```python
from build123d import *

# Parameters (mm, degrees)
SKETCH1_W           = 91
SKETCH1_H           = 104
SKETCH1_W_2         = 87
SKETCH1_H_2         = 100
BOSS_EXTRUDE1_DEPTH = 12
SKETCH2_W           = 91
SKETCH2_H           = 104
BOSS_EXTRUDE2_DEPTH = 2
SKETCH3_R           = 3.5
BOSS_EXTRUDE3_DEPTH = 12
SKETCH6_W           = 8
SKETCH6_H           = 5
BOSS_EXTRUDE4_DEPTH = 14
CUT_EXTRUDE1_REACH  = 141.879
SKETCH4_R           = 1.5
SKETCH7_R           = 2.9
CUT_EXTRUDE2_DEPTH  = 8
SKETCH8_W           = 33
SKETCH8_H           = 2
CUT_EXTRUDE3_DEPTH  = 1.3
SKETCH9_W           = 87.4
SKETCH9_H           = 100.4
SKETCH9_W_2         = 87
SKETCH9_H_2         = 100
CUT_EXTRUDE4_DEPTH  = 0.2
SKETCH10_W          = 6
SKETCH10_H          = 10
BOSS_EXTRUDE7_DEPTH = 5
CUT_EXTRUDE5_REACH  = 143.23
SKETCH11_R          = 0.75
SKETCH12_W          = 37
SKETCH12_H          = 7.6
CUT_EXTRUDE6_DEPTH  = 7
CUT_EXTRUDE7_REACH  = 142.975
SKETCH13_W          = 72
SKETCH13_H          = 7.6
FILLET1_R           = 10
FILLET2_R           = 2
SKETCH14_W          = 10
SKETCH14_H          = 4
CUT_EXTRUDE8_DEPTH  = 0.5


with BuildPart() as part:
    # Sketch1 → Boss-Extrude1 (new body)
    with BuildSketch(Plane(origin=(0, 0, 0), x_dir=(1, 0, 0), z_dir=(0, 1, 0))):
        with Locations((43.5, 50)):
            Rectangle(SKETCH1_W, SKETCH1_H)
        with Locations((43.5, 50)):
            Rectangle(SKETCH1_W_2, SKETCH1_H_2, mode=Mode.SUBTRACT)
    extrude(amount=-BOSS_EXTRUDE1_DEPTH)

    # Sketch2 → Boss-Extrude2 (add)
    with BuildSketch(Plane(origin=(0, 0, 0), x_dir=(1, 0, 0), z_dir=(0, 1, 0))):
        with Locations((43.5, 50)):
            Rectangle(SKETCH2_W, SKETCH2_H)
    extrude(amount=BOSS_EXTRUDE2_DEPTH)

    # Sketch3 → Boss-Extrude3 (add)
    with BuildSketch(Plane.XZ):
        with Locations(Location((5, -5, 0), (0, 0, 90))):
            Circle(SKETCH3_R)
        with Locations(Location((5, -95, 0), (0, 0, 90))):
            Circle(SKETCH3_R)
        with Locations(Location((50.38, -8.15, 0), (0, 0, 90))):
            Circle(SKETCH3_R)
        with Locations(Location((25, -50, 0), (0, 0, 90))):
            Circle(SKETCH3_R)
    extrude(amount=BOSS_EXTRUDE3_DEPTH)

    # Sketch6 → Boss-Extrude4 (add, through all)
    with BuildSketch(Plane(origin=(0, 2, 0), x_dir=(1, 0, 0), z_dir=(0, 1, 0))):
        with Locations((85, 104.5)):
            Rectangle(SKETCH6_W, SKETCH6_H)
        with Locations((85, -4.5)):
            Rectangle(SKETCH6_W, SKETCH6_H)
    extrude(amount=-BOSS_EXTRUDE4_DEPTH)

    # Sketch4 → Cut-Extrude1 (cut, up to next)
    with BuildSketch(Plane(origin=(0, 2, 0), x_dir=(1, 0, 0), z_dir=(0, 1, 0)), mode=Mode.PRIVATE) as cut_extrude1_sk1:
        with Locations(Location((5, 5, 0), (0, 0, 270))):
            Circle(SKETCH4_R)
    cut_extrude1_tool1 = extrude(cut_extrude1_sk1.sketch, amount=-CUT_EXTRUDE1_REACH, mode=Mode.PRIVATE) & part.part
    # Sketch4 → Cut-Extrude1 (cut, up to next)
    with BuildSketch(Plane(origin=(0, 2, 0), x_dir=(1, 0, 0), z_dir=(0, 1, 0)), mode=Mode.PRIVATE) as cut_extrude1_sk2:
        with Locations(Location((5, 95, 0), (0, 0, 270))):
            Circle(SKETCH4_R)
    cut_extrude1_tool2 = extrude(cut_extrude1_sk2.sketch, amount=-CUT_EXTRUDE1_REACH, mode=Mode.PRIVATE) & part.part
    # Sketch4 → Cut-Extrude1 (cut, up to next)
    with BuildSketch(Plane(origin=(0, 2, 0), x_dir=(1, 0, 0), z_dir=(0, 1, 0)), mode=Mode.PRIVATE) as cut_extrude1_sk3:
        with Locations(Location((50.38, 8.15, 0), (0, 0, 270))):
            Circle(SKETCH4_R)
    cut_extrude1_tool3 = extrude(cut_extrude1_sk3.sketch, amount=-CUT_EXTRUDE1_REACH, mode=Mode.PRIVATE) & part.part
    # Sketch4 → Cut-Extrude1 (cut, up to next)
    with BuildSketch(Plane(origin=(0, 2, 0), x_dir=(1, 0, 0), z_dir=(0, 1, 0)), mode=Mode.PRIVATE) as cut_extrude1_sk4:
        with Locations(Location((25, 50, 0), (0, 0, 270))):
            Circle(SKETCH4_R)
    cut_extrude1_tool4 = extrude(cut_extrude1_sk4.sketch, amount=-CUT_EXTRUDE1_REACH, mode=Mode.PRIVATE) & part.part
    # Sketch4 → Cut-Extrude1 (cut, up to next)
    with BuildSketch(Plane(origin=(0, 2, 0), x_dir=(1, 0, 0), z_dir=(0, 1, 0)), mode=Mode.PRIVATE) as cut_extrude1_sk5:
        with Locations(Location((85, 103.5, 0), (0, 0, 270))):
            Circle(SKETCH4_R)
    cut_extrude1_tool5 = extrude(cut_extrude1_sk5.sketch, amount=-CUT_EXTRUDE1_REACH, mode=Mode.PRIVATE) & part.part
    # Sketch4 → Cut-Extrude1 (cut, up to next)
    with BuildSketch(Plane(origin=(0, 2, 0), x_dir=(1, 0, 0), z_dir=(0, 1, 0)), mode=Mode.PRIVATE) as cut_extrude1_sk6:
        with Locations(Location((85, -3.5, 0), (0, 0, 270))):
            Circle(SKETCH4_R)
    cut_extrude1_tool6 = extrude(cut_extrude1_sk6.sketch, amount=-CUT_EXTRUDE1_REACH, mode=Mode.PRIVATE) & part.part
    add(cut_extrude1_tool1.solids().sort_by_distance((5, 2, -5))[0], mode=Mode.SUBTRACT)
    add(cut_extrude1_tool2.solids().sort_by_distance((5, 2, -95))[0], mode=Mode.SUBTRACT)
    add(cut_extrude1_tool3.solids().sort_by_distance((50.38, 2, -8.15))[0], mode=Mode.SUBTRACT)
    add(cut_extrude1_tool4.solids().sort_by_distance((25, 2, -50))[0], mode=Mode.SUBTRACT)
    add(cut_extrude1_tool5.solids().sort_by_distance((85, 2, -103.5))[0], mode=Mode.SUBTRACT)
    add(cut_extrude1_tool6.solids().sort_by_distance((85, 2, 3.5))[0], mode=Mode.SUBTRACT)

    # Sketch7 → Cut-Extrude2 (cut)
    with BuildSketch(Plane(origin=(0, 2, 0), x_dir=(1, 0, 0), z_dir=(0, 1, 0))):
        with Locations(Location((5, 5, 0), (0, 0, 270))):
            Circle(SKETCH7_R)
        with Locations(Location((25, 50, 0), (0, 0, 270))):
            Circle(SKETCH7_R)
        with Locations(Location((50.38, 8.15, 0), (0, 0, 270))):
            Circle(SKETCH7_R)
        with Locations(Location((5, 95, 0), (0, 0, 270))):
            Circle(SKETCH7_R)
        with Locations(Location((85, 103.5, 0), (0, 0, 270))):
            Circle(SKETCH7_R)
        with Locations(Location((85, -3.5, 0), (0, 0, 270))):
            Circle(SKETCH7_R)
    extrude(amount=-CUT_EXTRUDE2_DEPTH, mode=Mode.SUBTRACT)

    # Sketch8 → Cut-Extrude3 (cut)
    with BuildSketch(Plane.XY.offset(-100)):
        with Locations((66.5, -11)):
            Rectangle(SKETCH8_W, SKETCH8_H)
    extrude(amount=-CUT_EXTRUDE3_DEPTH, mode=Mode.SUBTRACT)

    # Sketch9 → Cut-Extrude4 (cut)
    with BuildSketch(Plane(origin=(0, -12, 0), x_dir=(-1, 0, 0), z_dir=(0, -1, 0))):
        with Locations((-43.5, 50)):
            Rectangle(SKETCH9_W, SKETCH9_H)
        with Locations((-43.5, 50)):
            Rectangle(SKETCH9_W_2, SKETCH9_H_2, mode=Mode.SUBTRACT)
    extrude(amount=-CUT_EXTRUDE4_DEPTH, mode=Mode.SUBTRACT)

    # Sketch10 → Boss-Extrude7 (add)
    with BuildSketch(Plane.XY.offset(-100)):
        with Locations((53, -5)):
            Rectangle(SKETCH10_W, SKETCH10_H)
        with Locations((80, -5)):
            Rectangle(SKETCH10_W, SKETCH10_H)
    extrude(amount=BOSS_EXTRUDE7_DEPTH)

    # Sketch11 → Cut-Extrude5 (cut, up to next)
    with BuildSketch(Plane(origin=(0, 0, -102), x_dir=(-1, 0, 0), z_dir=(0, 0, -1)), mode=Mode.PRIVATE) as cut_extrude5_sk1:
        with Locations((-43.257, -10.5)):
            Circle(SKETCH11_R)
    cut_extrude5_tool1 = extrude(cut_extrude5_sk1.sketch, amount=-CUT_EXTRUDE5_REACH, mode=Mode.PRIVATE) & part.part
    # Sketch11 → Cut-Extrude5 (cut, up to next)
    with BuildSketch(Plane(origin=(0, 0, -102), x_dir=(-1, 0, 0), z_dir=(0, 0, -1)), mode=Mode.PRIVATE) as cut_extrude5_sk2:
        with BuildLine():
            Line((-41.957, -12), (-31.457, -12))
            Line((-31.457, -12), (-31.457, -9))
            ThreePointArc((-31.457, -9), (-31.749893219, -8.292893219), (-32.457, -8))
            Line((-32.457, -8), (-40.957, -8))
            ThreePointArc((-40.957, -8), (-41.664106781, -8.292893219), (-41.957, -9))
            Line((-41.957, -9), (-41.957, -12))
        make_face()
    cut_extrude5_tool2 = extrude(cut_extrude5_sk2.sketch, amount=-CUT_EXTRUDE5_REACH, mode=Mode.PRIVATE) & part.part
    add(cut_extrude5_tool1.solids().sort_by_distance((43.257, -10.5, -102))[0], mode=Mode.SUBTRACT)
    add(cut_extrude5_tool2.solids().sort_by_distance((36.707, -10.018343, -102))[0], mode=Mode.SUBTRACT)

    # Sketch12 → Cut-Extrude6 (cut)
    with BuildSketch(Plane.XY.offset(2)):
        with Locations((32.85, -8.2)):
            Rectangle(SKETCH12_W, SKETCH12_H)
    extrude(amount=-CUT_EXTRUDE6_DEPTH, mode=Mode.SUBTRACT)

    # Sketch13 → Cut-Extrude7 (cut, up to next)
    with BuildSketch(Plane.ZY.offset(2), mode=Mode.PRIVATE) as cut_extrude7_sk1:
        with Locations((-50, -8.2)):
            Rectangle(SKETCH13_W, SKETCH13_H)
    cut_extrude7_tool1 = extrude(cut_extrude7_sk1.sketch, amount=-CUT_EXTRUDE7_REACH, mode=Mode.PRIVATE) & part.part
    add(cut_extrude7_tool1.solids().sort_by_distance((-2, -8.2, -50))[0], mode=Mode.SUBTRACT)

    # Fillet1
    # the kernel refuses this fillet: 10 mm, written as the material it adds along each edge
    with BuildSketch(Plane(origin=(81, 2, -102), x_dir=(0, 0, -1), z_dir=(0, -1, 0))) as fillet1_piece_1:
        with BuildLine():
            CenterArc((10, -8.660254038), FILLET1_R, 120, 60)
            Line((0, -8.660254038), (-0.2, -8.660254038))
            Line((-0.2, -8.660254038), (-0.2, 0))
            Line((-0.2, 0), (0, 0.2))
            ThreePointArc((0, 0.2), (2.5, 0.2), (4.9, 0.173205081))
            Line((4.9, 0.173205081), (5, 0))
        make_face()
    extrude(amount=14)
    with BuildSketch(Plane(origin=(81, 2, 2), x_dir=(-1, 0, 0), z_dir=(0, -1, 0))) as fillet1_piece_2:
        with BuildLine():
            CenterArc((8.660254038, -10), FILLET1_R, 90, 60)
            Line((0, -5), (-0.173205081, -4.9))
            ThreePointArc((-0.173205081, -4.9), (-0.2, -2.5), (-0.2, 0))
            Line((-0.2, 0), (0, 0.2))
            Line((0, 0.2), (8.660254038, 0.2))
            Line((8.660254038, 0.2), (8.660254038, 0))
        make_face()
    extrude(amount=14)

    # Fillet2
    fillet2_edges = [part.edges().sort_by_distance(p)[0] for p in [
        (81, -5, -107),
        (89, -5, -107),
        (89, -5, 7),
        (81, -5, 7),
        (-2, -5, 2),
        (-2, -5, -102),
    ]]
    fillet(fillet2_edges, radius=FILLET2_R)

    # Sketch14 → Cut-Extrude8 (cut)
    with BuildSketch(Plane.XY.offset(-100)):
        with Locations((21.757, -10)):
            Rectangle(SKETCH14_W, SKETCH14_H)
    extrude(amount=-CUT_EXTRUDE8_DEPTH, mode=Mode.SUBTRACT)


solid = part.part
```
The model under review builds one solid part; all positions refer to its coordinate system, in mm. A direction names the side the tool comes from. Give positions to 0.01 mm unless a question says otherwise; leave off trailing zeros. Order: outer loops, then holes, each group sorted by start corner. A loop starts at its lowest first (then second) coordinate and runs counter-clockwise, first axis right, second up. Notation, with made-up numbers: (-35, 28.5) - (5, 28.5) arc R14 ccw to (5, 45.5) - close; hole circle Ø8 at (47, 4.25). An arc over 180 degrees is marked (long way). Use CSV: the item, a comma, the result in double quotes. Start each with the question number.
Q1. Clearance check with flat-ended pins moving along their axes: pin 1 Ø1.2 at (x, y) = (23, -10) entering from +Z; pin 2 Ø1.8 at (x, z) = (5, -95) entering from -Y; pin 3 Ø6 at (x, y) = (61.5, -3) entering from -Z; pin 4 Ø0.6 at (x, y) = (58.5, -10.5) entering from +Z. State where each tip first meets the part, or that it passes through.
Q2. We need section B-B, the plane z = -50. Write out the cut boundary in (x, y), and give its area (3 significant figures).
Q3. To check wall thickness, follow line 1 along X through (y, z) = (-1.75, -50); line 2 along X through (y, z) = (-1, -8.15); line 3 along Z through (x, y) = (42, -3.5). State the ranges of each line that lie inside material, in increasing order. Write a range as [from, to].
Q4. The part is to be moulded in two halves that separate along X. For faces 4 (the cylindrical face through (23.89, -1.94, -47.32)), 5 (the flat face through (85, -5, -107)), say which applies: +X half, -X half, draft (parallel to the pull), parting line (faces both ways), or undercut.
Q5. We need section A-A, the plane x = 85. Write out the cut boundary in (y, z), and give its area (3 significant figures).
Q6. We need section C-C, the plane x = 25. Write out the cut boundary in (y, z).
Q7. We need section D-D, the plane z = -81.5. Write out the cut boundary in (x, y), and give its area (3 significant figures).
Q8. Tool access review of faces 1 (the flat face through (36, -4, 2)), 2 (the flat face through (84, -6, 5)), 3 (the flat face through (0, -3, -49)): name each direction out of +Z, -Z, +X, -X, +Y, -Y from which nothing blocks a thin tool from reaching the whole face with its end or side.
Outcome:
1,pin 1,"stops at z = -46.79"
1,pin 2,"passes through"
1,pin 3,"stops at z = -102"
1,pin 4,"stops at z = 2"
2,outline,"(-2, -4.4) - (0, -4.4) - (0, 0) - (21.5, 0) - (21.5, -12) - (23.5, -12) - (23.5, -6) - (22.1, -6) - (22.1, 2) - (-2, 2) - close; (26.5, -12) - (28.5, -12) - (28.5, 0) - (87, 0) - (87, -11.8) - (87.2, -11.8) - (87.2, -12) - (89, -12) - (89, 2) - (27.9, 2) - (27.9, -6) - (26.5, -6) - close"
2,area,"234 mm^2"
3,line 1,"x = [-2, 0], [21.5, 22.1], [27.9, 28.5], [87, 89]"
3,line 2,"x = [-2, 0], [3.47, 6.53], [46.88, 47.48], [53.28, 53.88], [87, 89]"
3,line 3,"z = [-102, -100], [0, 2]"
4,face 4,"undercut"
4,face 5,"draft"
5,outline,"(-12, -107) - (2, -107) - (2, -106.4) - (-6, -106.4) - (-6, -105) - (-12, -105) - close; (-12, -102) - (-6, -102) - (-6, -100.6) - (2, -100.6) - (2, 0.6) - (-6, 0.6) - (-6, 2) - (-12, 2) - (-12, 0.2) - (-11.8, 0.2) - (-11.8, 0) - (0, 0) - (0, -100) - (-11.8, -100) - (-11.8, -100.2) - (-12, -100.2) - close; (-12, 5) - (-6, 5) - (-6, 6.4) - (2, 6.4) - (2, 7) - (-12, 7) - close"
5,area,"267 mm^2"
6,outline,"(-12, -102) - (2, -102) - (2, -52.9) - (-6, -52.9) - (-6, -51.5) - (-12, -51.5) - (-12, -53.5) - (0, -53.5) - (0, -100) - (-8, -100) - (-8, -100.5) - (-12, -100.5) - close; (-12, -48.5) - (-6, -48.5) - (-6, -47.1) - (2, -47.1) - (2, 2) - (-4.4, 2) - (-4.4, 0) - (0, 0) - (0, -46.5) - (-12, -46.5) - close"
7,outline,"(-2, -4.4) - (0, -4.4) - (0, 0) - (87, 0) - (87, -11.8) - (87.2, -11.8) - (87.2, -12) - (89, -12) - (89, 2) - (-2, 2) - close"
7,area,"215 mm^2"
8,face 1,"+Z, -X, +Y, -Y"
8,face 2,"+Y"
8,face 3,"-Y"
